```python
from build123d import *

# Parameters (mm, degrees)
SKETCH1_W           = 23.2
SKETCH1_H           = 22.8
SKETCH1_W_2         = 4
SKETCH1_H_2         = 5
BOSS_EXTRUDE1_DEPTH = 1.6
SKETCH1_4_W         = 4
SKETCH1_4_H         = 5
BOSS_EXTRUDE2_DEPTH = 3.15
FILLET1_R           = 2.5
SKETCH2_R           = 1.75
CUT_EXTRUDE1_DEPTH  = 3.1
SKETCH3_W           = 2.5
SKETCH3_H           = 10
SKETCH3_H_2         = 7.5
BOSS_EXTRUDE3_DEPTH = 2.6
SKETCH4_W           = 0.6
SKETCH4_H           = 0.6
BOSS_EXTRUDE4_DEPTH = 5


with BuildPart() as part:
    # Sketch1 → Boss-Extrude1 (new body)
    with BuildSketch(Plane(origin=(0, 0, 0), x_dir=(1, 0, 0), z_dir=(0, 1, 0))):
        Rectangle(SKETCH1_W, SKETCH1_H)
        Rectangle(SKETCH1_W_2, SKETCH1_H_2, mode=Mode.SUBTRACT)
    extrude(amount=BOSS_EXTRUDE1_DEPTH)

    # Sketch1_4 → Boss-Extrude2 (add)
    with BuildSketch(Plane(origin=(0, 0, 0), x_dir=(1, 0, 0), z_dir=(0, 1, 0))):
        Rectangle(SKETCH1_4_W, SKETCH1_4_H)
    extrude(amount=BOSS_EXTRUDE2_DEPTH)

    # Fillet1
    fillet1_edges = [part.edges().sort_by_distance(p)[0] for p in [
        (-11.6, 0.8, 11.4),
        (-11.6, 0.8, -11.4),
        (11.6, 0.8, -11.4),
        (11.6, 0.8, 11.4),
    ]]
    fillet(fillet1_edges, radius=FILLET1_R)

    # Sketch2 → Cut-Extrude1 (cut)
    with BuildSketch(Plane(origin=(0, 1.6, 0), x_dir=(1, 0, 0), z_dir=(0, 1, 0))):
        with Locations(Location((-7.85, -7.65, 0), (0, 0, 270))):
            Circle(SKETCH2_R)
        with Locations(Location((-7.85, 7.65, 0), (0, 0, 270))):
            Circle(SKETCH2_R)
        with Locations(Location((7.85, -7.65, 0), (0, 0, 270))):
            Circle(SKETCH2_R)
        with Locations(Location((7.85, 7.65, 0), (0, 0, 270))):
            Circle(SKETCH2_R)
    extrude(amount=-CUT_EXTRUDE1_DEPTH, mode=Mode.SUBTRACT)

    # Sketch3 → Boss-Extrude3 (add)
    with BuildSketch(Plane.XZ):
        with Locations((6.85, -0.4)):
            Rectangle(SKETCH3_W, SKETCH3_H)
        with Locations((-6.85, -0.15)):
            Rectangle(SKETCH3_W, SKETCH3_H_2)
    extrude(amount=BOSS_EXTRUDE3_DEPTH)

    # Sketch4 → Boss-Extrude4 (add)
    with BuildSketch(Plane.XZ.offset(2.6)):
        with Locations((-6.85, -0.15)):
            Rectangle(SKETCH4_W, SKETCH4_H)
        with Locations((-6.85, 2.35)):
            Rectangle(SKETCH4_W, SKETCH4_H)
        with Locations((-6.85, -2.65)):
            Rectangle(SKETCH4_W, SKETCH4_H)
        with Locations((6.85, 3.35)):
            Rectangle(SKETCH4_W, SKETCH4_H)
        with Locations((6.85, 0.85)):
            Rectangle(SKETCH4_W, SKETCH4_H)
        with Locations((6.85, -1.65)):
            Rectangle(SKETCH4_W, SKETCH4_H)
        with Locations((6.85, -4.15)):
            Rectangle(SKETCH4_W, SKETCH4_H)
    extrude(amount=BOSS_EXTRUDE4_DEPTH)


solid = part.part
```
Verification items for the finished model (mm, model axes). A direction names the side the tool comes from. Give positions to 0.01 mm unless a question says otherwise; leave off trailing zeros. Order: outer loops, then holes, each group sorted by start corner. A loop starts at its lowest first (then second) coordinate and runs counter-clockwise, first axis right, second up. Notation, with made-up numbers: (-17.5, -33.75) - (33.5, -33.75) arc R25 ccw to (33.5, 2.25) - close; hole circle Ø5 at (-35, -4). An arc over 180 degrees is marked (long way). Answer as CSV lines item,"result". Start each with the question number.
Item 1: Section check B-B, the plane z = -8. Record the boundary of the cut face in (x, y).
Item 2: Section check A-A, the plane y = -6. Record the boundary of the cut face in (x, z).
Item 3: Mould release check, pull along Z, two halves, no side actions. Record for faces 4 (the face through (2, 2, 0)), 5 (the face through (-8.91, 0.81, -9.04)), 6 (the face through (-10.887, 0.811, -10.648)): released by +Z, released by -Z, zero draft, split by the parting line, or undercut.
Item 4: Section check D-D, the plane y = -0.5. Record the boundary of the cut face in (x, z), plus the area to 4 significant figures.
Item 5: Material ranges on L1, parallel to Z at x = -6.75, y = -3.25; L2, parallel to X at y = 0.85, z = 7.65; L3, parallel to X at y = -0.75, z = -0.75, recorded low to high.
Item 6: Gauge pin test, flat ends, axial feed: pin 1 (0.5 mm diameter, centred on y = -5, z = 0, fed in from +X); pin 2 (1.3 mm diameter, centred on y = -1, z = -0.5, fed in from +X); pin 3 (0.5 mm diameter, centred on y = -5, z = -4, fed in from +X). Record the tip position at first contact, or that the pin passes through.
Item 7: Access from +Z, -Z, +X, -X, +Y, -Y to the whole of each face (thin tool, end or side, straight path). Record for faces 1 (the face through (8.1, -1, 0)), 2 (the face through (0, 2, -2.5)), 3 (the face through (-5.6, -1, 0)).
Item 8: Section check C-C, the plane x = 8.5. Record the boundary of the cut face in (y, z), plus the area to 3 significant figures.
Filled in:
1,outline,"(-11.6, 0) - (-9.56, 0) - (-9.56, 1.6) - (-11.6, 1.6) - close; (-6.14, 0) - (6.14, 0) - (6.14, 1.6) - (-6.14, 1.6) - close; (9.56, 0) - (11.6, 0) - (11.6, 1.6) - (9.56, 1.6) - close"
2,outline,"(-7.15, -2.95) - (-6.55, -2.95) - (-6.55, -2.35) - (-7.15, -2.35) - close; (-7.15, -0.45) - (-6.55, -0.45) - (-6.55, 0.15) - (-7.15, 0.15) - close; (-7.15, 2.05) - (-6.55, 2.05) - (-6.55, 2.65) - (-7.15, 2.65) - close; (6.55, -4.45) - (7.15, -4.45) - (7.15, -3.85) - (6.55, -3.85) - close; (6.55, -1.95) - (7.15, -1.95) - (7.15, -1.35) - (6.55, -1.35) - close; (6.55, 0.55) - (7.15, 0.55) - (7.15, 1.15) - (6.55, 1.15) - close; (6.55, 3.05) - (7.15, 3.05) - (7.15, 3.65) - (6.55, 3.65) - close"
3,face 4,"zero draft"
3,face 5,"undercut"
3,face 6,"released by -Z"
4,outline,"(-8.1, -3.9) - (-5.6, -3.9) - (-5.6, 3.6) - (-8.1, 3.6) - close; (5.6, -5.4) - (8.1, -5.4) - (8.1, 4.6) - (5.6, 4.6) - close"
4,area,"43.75 mm^2"
5,L1,"-2.95 to -2.35, -0.45 to 0.15, 2.05 to 2.65"
5,L2,"-11.6 to -9.6, -6.1 to 6.1, 9.6 to 11.6"
5,L3,"-8.1 to -5.6, 5.6 to 8.1"
6,pin 1,"x = -6.55"
6,pin 2,"x = 8.1"
6,pin 3,"x = 7.15"
7,face 1,"+Z, -Z, +X, -Y"
7,face 2,"-Z, +X, -X, +Y"
7,face 3,"+Z, -Z, -Y"
8,outline,"(0, -11.4) - (1.6, -11.4) - (1.6, -9.27) - (0, -9.27) - close; (0, -6.03) - (1.6, -6.03) - (1.6, 6.03) - (0, 6.03) - close; (0, 9.27) - (1.6, 9.27) - (1.6, 11.4) - (0, 11.4) - close"
8,area,"26.1 mm^2"
